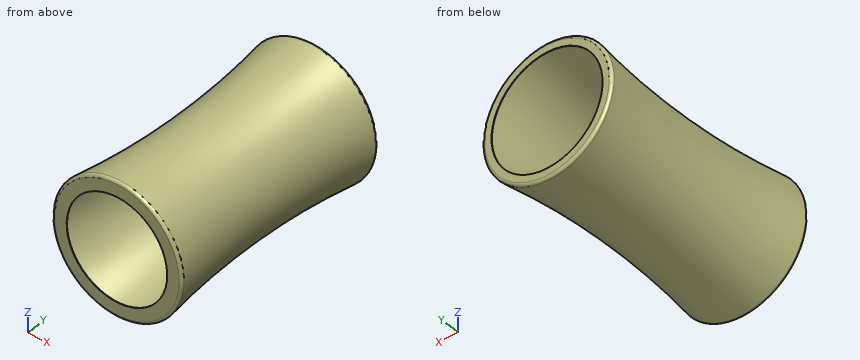
```python
from build123d import *


with BuildPart() as part:
    # Sketch1 → Revolve1 (revolve)
    with BuildSketch(Plane.XY, mode=Mode.PRIVATE) as revolve1_sk:
        with BuildLine():
            Line((12.5, -114.686619696), (12.5, -114.786619696))
            Line((12.5, -114.786619696), (14.004531695, -114.786619696))
            ThreePointArc((14.004531695, -114.786619696), (14.357864572, -114.932974966), (14.504219842, -115.286307843))
            ThreePointArc((14.504219842, -115.286307843), (12.706614743, -140.661619696), (14.504219842, -166.036931549))
            ThreePointArc((14.504219842, -166.036931549), (14.357864572, -166.390264426), (14.004531695, -166.536619696))
            Line((14.004531695, -166.536619696), (11.318941473, -166.536619696))
            Line((11.318941473, -166.536619696), (11.318941473, -166.636619696))
            Line((11.318941473, -166.636619696), (14.004531695, -166.636619696))
            ThreePointArc((14.004531695, -166.636619696), (14.42857525, -166.460975104), (14.604219842, -166.036931549))
            ThreePointArc((14.604219842, -166.036931549), (12.805615521, -140.661619696), (14.604219842, -115.286307843))
            ThreePointArc((14.604219842, -115.286307843), (14.42857525, -114.862264288), (14.004531695, -114.686619696))
            Line((14.004531695, -114.686619696), (12.5, -114.686619696))
        make_face()
    revolve(revolve1_sk.sketch.rotate(Axis((0, 0, 0), (0, -1, 0)), 90), axis=Axis((0, 0, 0), (0, -1, 0)))


solid = part.part
```
Here's how the part is built. I have some questions about the finished solid (model axes, mm). Coordinates: 2 decimals unless noted, no trailing zeros. Loops run counter-clockwise (first coordinate to the right, second up) from the corner with the lowest first, then second, coordinate; pieces in that order, holes last. Notation, with made-up numbers: (51, 21) - (79, 21) arc R30 cw to (79, 48) - close; hole circle Ø8 at (73, 47). An arc over 180 degrees is marked (long way). Answer as CSV lines item,"result".
Q1. If we section it at D-D, the plane y = -135.5: Write out the boundary of the cut face in (x, z).
Response:
outline,"circle Ø25.76 at (0, 0); hole circle Ø25.56 at (0, 0)"
Q2. If I drill on L1, parallel to Z at x = -11.75, y = -127; L2, parallel to Z at x = 11.75, y = -155.5, over which ranges is the centre line in solid material (lowest first)? Write a range as [from, to].
Response:
L1,"[-6.28, -6.07], [6.07, 6.28]"
L2,"[-6.48, -6.27], [6.27, 6.48]"
Q3. If we section it at C-C, the plane y = -151: Write out the boundary of the cut face in (x, z).
Response:
outline,"circle Ø26.21 at (0, 0); hole circle Ø26.01 at (0, 0)"
Q4. For pin 1 (2 mm diameter, centred on y = -145.5, z = -7.5, fed in from -X); pin 2 (4 mm diameter, centred on y = -158, z = -1, fed in from +X); pin 3 (15 mm diameter, centred on x = 0, z = 0, fed in from +Y); pin 4 (4 mm diameter, centred on y = -149, z = 7, fed in from -X), each with a flat end and sliding along its axis, tell me the tip position at first contact or that it passes through.
Response:
pin 1,"x = -11.11"
pin 2,"x = 13.83"
pin 3,"through"
pin 4,"x = -12.01"
Q5. If we section it at B-B, the plane x = 0: Write out the boundary of the cut face in (y, z).
Response:
outline,"(-166.64, -14) arc R0.6 ccw to (-166.04, -14.6) arc R179.9 cw to (-115.29, -14.6) arc R0.6 ccw to (-114.69, -14) - (-114.69, -12.5) - (-114.79, -12.5) - (-114.79, -14) arc R0.5 cw to (-115.29, -14.5) arc R180 ccw to (-166.04, -14.5) arc R0.5 cw to (-166.54, -14) - (-166.54, -11.32) - (-166.64, -11.32) - close; (-166.64, 11.32) - (-166.54, 11.32) - (-166.54, 14) arc R0.5 cw to (-166.04, 14.5) arc R180 ccw to (-115.29, 14.5) arc R0.5 cw to (-114.79, 14) - (-114.79, 12.5) - (-114.69, 12.5) - (-114.69, 14) arc R0.6 ccw to (-115.29, 14.6) arc R179.9 cw to (-166.04, 14.6) arc R0.6 ccw to (-166.64, 14) - close"
Q6. If we section it at A-A, the plane z = 0: Write out the boundary of the cut face in (x, y).
Response:
outline,"(-14.6, -166.04) arc R0.6 ccw to (-14, -166.64) - (-11.32, -166.64) - (-11.32, -166.54) - (-14, -166.54) arc R0.5 cw to (-14.5, -166.04) arc R180 ccw to (-14.5, -115.29) arc R0.5 cw to (-14, -114.79) - (-12.5, -114.79) - (-12.5, -114.69) - (-14, -114.69) arc R0.6 ccw to (-14.6, -115.29) arc R179.9 cw to start; (11.32, -166.64) - (14, -166.64) arc R0.6 ccw to (14.6, -166.04) arc R179.9 cw to (14.6, -115.29) arc R0.6 ccw to (14, -114.69) - (12.5, -114.69) - (12.5, -114.79) - (14, -114.79) arc R0.5 cw to (14.5, -115.29) arc R180 ccw to (14.5, -166.04) arc R0.5 cw to (14, -166.54) - (11.32, -166.54) - close"
